```python
from build123d import *

# Parameters (mm, degrees)
BOSS_EXTRUDE1_DEPTH = 57
FILLET1_R           = 15


with BuildPart() as part:
    # Sketch1 → Boss-Extrude1 (new body)
    with BuildSketch(Plane.XY):
        with BuildLine():
            Line((65, 0), (0, 0))
            add(Edge.make_bspline(
                [(0, 0), (-3.420787062, 3.445195102), (-7.060889651, 4.793606126), (-10.827974412, 5)],
                knots=[0, 0, 0, 0, 0.227402819, 0.227402819, 0.227402819, 0.227402819], degree=3))
            Line((-10.827974412, 5), (-12.998410552, 5))
            add(Edge.make_bspline(
                [(-12.998410552, 5), (-25.222609251, 4.375360382), (-38.571253465, -6.117915944), (-50, 5)],
                knots=[0.270809768, 0.270809768, 0.270809768, 0.270809768, 1, 1, 1, 1], degree=3))
            Line((-50, 5), (-50, 0))
            add(Edge.make_bspline(
                [(0, -5), (-14.762430124, 10.348316204), (-34.295343775, -15.48284378), (-50, 0)],
                knots=[0, 0, 0, 0, 1, 1, 1, 1], degree=3))
            Line((0, -5), (65, -5))
            Line((65, -5), (65, 0))
        make_face()
        with BuildLine():
            Line((80, 0), (65, 0))
            Line((65, 0), (65, -5))
            add(Edge.make_bspline(
                [(65, -5), (72.93083611, -3.380904469), (80, 0)],
                knots=[0, 0, 0, 0.467251417, 0.467251417, 0.467251417], degree=2))
        make_face()
        with BuildLine():
            add(Edge.make_bspline(
                [(65, 0), (81.973380543, 3.465148466), (95, 15)],
                knots=[0, 0, 0, 1, 1, 1], degree=2))
            Line((65, 0), (80, 0))
            add(Edge.make_bspline(
                [(80, 0), (88.060086943, 3.85482419), (95, 10)],
                knots=[0.467251417, 0.467251417, 0.467251417, 1, 1, 1], degree=2))
            Line((95, 10), (95, 15))
        make_face()
    extrude(amount=BOSS_EXTRUDE1_DEPTH)

    # Fillet1
    fillet1_edges = [part.edges().sort_by_distance(p)[0] for p in [
        (0, -5, 28.5),
    ]]
    fillet(fillet1_edges, radius=FILLET1_R)


solid = part.part
```
Read the model definition and answer for the solid it produces. Units are mm, in the model's axes. A direction names the side the tool comes from. Coordinates: 2 decimals unless noted, no trailing zeros. Order: outer loops, then holes, each group sorted by start corner. A loop starts at its lowest first (then second) coordinate and runs counter-clockwise, first axis right, second up. Notation, with made-up numbers: (5.25, 54.5) - (57.25, 54.5) arc R28 cw to (57.25, 81.5) - close; hole circle Ø6 at (-16.75, 82). An arc over 180 degrees is marked (long way). Answer as a JSON object with one key per item and string values. Group by question number.
Item 1: Consider probe 1 along Y at (x, z) = (27.5, 3.5); probe 2 along Y at (x, z) = (-35, 38.5); probe 3 along X at (y, z) = (8.25, 50.5). Determine where each line is inside the solid, lowest interval first. Write a range as from..to.
Item 2: A tool of negligible diameter and unlimited length cuts with its end or side. For faces 1 (the face through (33, 0, 28)), 2 (the face through (95, 12, 28)), 3 (the face through (35, -5, 28)), from which of +Z, -Z, +X, -X, +Y, -Y can it reach the whole face along a straight path? Write none if from no direction.
Item 3: Section A-A (y = 2.5) is taken. State how many separate pieces and enclosed holes the cut face has, plus the area to 3 significant figures.
Item 4: Section B-B (x = 41) is taken. Give the vertices of the cut face in (y, z), plus the area to 3 significant figures.
Item 5: Flat-ended cylindrical pins translate along their axes: P1, Ø3, axis at y = 6.5, z = 12.5, coming from the +X side; P2, Ø8, axis at x = 12.5, z = 26, coming from the -Y side; P3, Ø1, axis at x = -7, z = 16, coming from the +Y side. Find the tip coordinate at first contact, or state that the pin passes through.
Results are:
{
 "1": {"probe 1": "y = -5..0", "probe 2": "y = -5..0.07", "probe 3": "x = 85.95..92.94"},
 "2": {"face 1": "+Z, -Z, +Y", "face 2": "+Z, -Z, +X, +Y, -Y", "face 3": "+Z, -Z, +X, -Y"},
 "3": {"separate pieces": "3", "enclosed holes": "0", "area": "2,020 mm^2"},
 "4": {"outline": "(-5, 0) - (0, 0) - (0, 57) - (-5, 57) - close", "area": "285 mm^2"},
 "5": {"P1": "stops at x = 92.64", "P2": "stops at y = -5", "P3": "stops at y = 4.49"}
}
